The listing builds one solid part. Answer for the finished solid, in the listing's coordinates (mm). Face numbers are marked on the shaded views. A direction names the side the tool comes from. Give positions to 0.01 mm unless a question says otherwise; leave off trailing zeros. Order: outer loops, then holes, each group sorted by start corner. A loop starts at its lowest first (then second) coordinate and runs counter-clockwise, first axis right, second up.
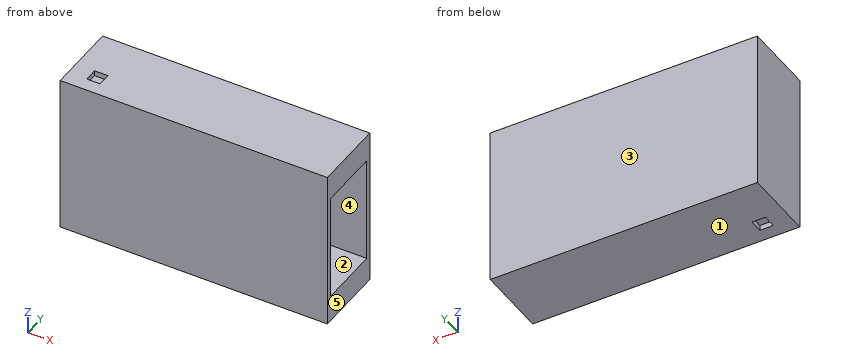
Autodesk Inventor part; units mm, degrees
ref_plane "XZ Plane" through (0, 0, 0) normal (0, 1, 0) x (-1, 0, 0)
ref_plane "XY Plane" through (0, 0, 0) normal (0, 0, 1) x (1, 0, 0)
sketch "Эскиз1" plane through (0, 0, 0) normal (1, 0, 0) x (0, 1, 0)
  line L0 (0, 0) -> (25, 0)
  line L1 (25, 0) -> (25, -60)
  line L2 (25, -60) -> (0, -60)
  line L3 (0, -60) -> (0, 0)
  line L4 (0, 0) -> (0, -2)
  line L5 (0, -2) -> (23, -2)
  line L6 (23, -2) -> (23, -58)
  line L7 (23, -58) -> (0, -58)
  line L8 (0, 0) -> (0, -10)
  line L9 (0, -10) -> (23, -10)
  line L10 (0, -10) -> (0, -50)
  line L11 (0, -50) -> (23, -50)
  line L12 (0, 0) -> (-2, 0)
  line L13 (-2, 0) -> (-2, -60)
  line L14 (-2, -60) -> (0, -60)
  line L15 (0, -10) -> (0, -50)
  dimension "d0" = 25
  dimension "d1" = 60
  dimension "d2" = 2
  dimension "d3" = 23
  dimension "d4" = 56
  dimension "d5" = 10
  dimension "d6" = 40
  dimension "d26" = 2
sketch "Эскиз2" plane through (0, 0, 0) normal (0, 0, 1) x (1, 0, 0)
  line L0 (0, 0) -> (0, 25)
  line L1 (0, 25) -> (-100, 25)
  line L2 (-100, 25) -> (-100, 0)
  line L3 (-100, 0) -> (0, 0)
  line L4 (-100, 0) -> (-98, 0)
  line L5 (-98, 0) -> (-98, 23)
  line L6 (-98, 23) -> (-2, 23)
  line L7 (-2, 23) -> (-2, 0)
  line L8 (-98, 0) -> (-93, 0)
  line L9 (-93, 3) -> (-88, 3)
  line L10 (-88, 3) -> (-88, 8)
  line L11 (-88, 8) -> (-93, 8)
  line L12 (-93, 8) -> (-93, 3)
  line L13 (0, 0) -> (0, -2)
  line L14 (0, -2) -> (-100, -2)
  line L15 (-100, -2) -> (-100, 0)
  line L16 (-98, 0) -> (-2, 0)
  dimension "d7" = 25
  dimension "d8" = 100
  dimension "d9" = 2
  dimension "d10" = 23
  dimension "d11" = 96
  dimension "d13" = 3
  dimension "d14" = 5
  dimension "d15" = 5
  dimension "d16" = 88
  dimension "d17" = 17
  dimension "d27" = 2
ref_plane "РабПлоскость3" through (-2, 0, 0) normal (1, 0, 0) x (0, 1, 0)
sketch "Эскиз3" plane through (-2, 0, 0) normal (1, 0, 0) x (0, 1, 0)
  line L0 (0, 0) -> (0, -2)
  line L1 (0, -2) -> (23, -2)
  line L2 (23, -2) -> (23, -58)
  line L3 (23, -58) -> (0, -58)
  line L4 (0, -58) -> (0, -50)
  line L5 (0, -50) -> (23, -50)
  line L6 (23, -50) -> (23, -10)
  line L7 (23, -10) -> (0, -10)
  line L8 (0, -10) -> (0, -2)
  line L9 (0, -50) -> (0, -58)
  dimension "d30" = 2
  dimension "d31" = 23
  dimension "d32" = 56
  dimension "d33" = 8
  dimension "d34" = 40
extrude "Выдавливание5" add sketch "Эскиз2" against normal blind 60 contours L3 L7 L6 L5 L2 L1 L0 | L3 L5 L6 L7
extrude "Выдавливание6" add sketch "Эскиз2" against normal blind 60 contours L13 L14 L15 L3
extrude "Выдавливание7" cut sketch "Эскиз1" against normal blind 98 contours L9 L6 L11 L3
extrude "Выдавливание8" add sketch "Эскиз3" against normal blind 98
1) Find section B-B (x = -76.5). Write down the section's boundary in (y, z).
Geometry says:
outline: (-2, -60) - (25, -60) - (25, 0) - (-2, 0) - close; hole (0, -50) - (23, -50) - (23, -10) - (0, -10) - close
2) For a pull along Z with two mould halves and no side action, classify the marked faces 1, 2 and 3 as +Z half, -Z half, draft (parallel to the pull), parting line (faces both ways), or undercut.
Geometry says:
face 1: -Z half
face 2: undercut
face 3: draft
3) Find section A-A (y = 13.5). Write down the section's boundary in (x, z), then the cut area to 3 significant figures.
Geometry says:
outline: (-100, -60) - (0, -60) - (0, -50) - (-98, -50) - (-98, -10) - (0, -10) - (0, 0) - (-100, 0) - close
area: 2,080 mm2
4) Find section C-C (z = -23.5). Write down the section's boundary in (x, y), then the cut area to 3 significant figures.
Geometry says:
outline: (-100, -2) - (0, -2) - (0, 0) - (-98, 0) - (-98, 23) - (0, 23) - (0, 25) - (-100, 25) - close
area: 446 mm2
5) Straight lines are drawn through the part: probe 1 along Y at (x, z) = (-27, -13); probe 2 along Z at (x, y) = (-18, 19.5); probe 3 along X at (y, z) = (20.25, -25.5). For each, find the intervals that lie inside material, in ascending order.
Geometry says:
probe 1: y = -2 to 0, 23 to 25
probe 2: z = -60 to -50, -10 to 0
probe 3: x = -100 to -98
6) Given P1, Ø7, axis at y = 10.5, z = -33.5, coming from the +X side; P2, Ø2.5, axis at x = -89.5, y = 6.5, coming from the -Z side, each flat-ended and moving along its own axis, determine where each tip first touches the part or whether it passes through.
Geometry says:
P1: stops at x = -98
P2: stops at z = -58
7) A tool of negligible diameter and unlimited length cuts with its end or side. For the marked faces 4 and 5, from which of +Z, -Z, +X, -X, +Y, -Y can it reach the whole face along a straight path? Write none if from no direction.
Geometry says:
face 4: +X
face 5: +Z, -Z, +X, +Y, -Y
8) Find section D-D (y = 5.5). Write down the section's boundary in (x, z), then the cut area to 3 significant figures.
Geometry says:
outline: (-100, -60) - (-93, -60) - (-93, -58) - (-88, -58) - (-88, -60) - (0, -60) - (0, -50) - (-98, -50) - (-98, -10) - (0, -10) - (0, 0) - (-88, 0) - (-88, -2) - (-93, -2) - (-93, 0) - (-100, 0) - close
area: 2,060 mm2
